The listing builds one solid part. Answer for the finished solid, in the listing's coordinates (mm). Face numbers are marked on the shaded views. A direction names the side the tool comes from. Round coordinates to 2 decimals unless told otherwise and drop trailing zeros. Write each loop counter-clockwise with the first axis right and the second up, starting at its lowest first coordinate (ties: lowest second). Pieces come first, ordered by that corner, then holes. Notation, with made-up numbers: (38.5, 30) - (56.5, 30) arc R15 ccw to (56.5, 58) - close; hole circle Ø4 at (2, 22). An arc over 180 degrees is marked (long way). Return JSON: item names as keys, results as strings. Group by question number.
from build123d import *

# Parameters (mm, degrees)
EXTRUDE_1_DEPTH          = 1
CUT_EXTRUDE_1_DEPTH      = 5
SKETCH_4_R               = 0.4
CUT_EXTRUDE_2_DEPTH      = 5
PATTERN_CIRCULAR_3_COUNT = 3
FILLET_1_R               = 0.4
FILLET_2_R               = 2


with BuildPart() as part:
    # 草图1 → 凸台-拉伸1 (new, symmetric)
    with BuildSketch(Plane(origin=(0, 0, 0), x_dir=(1, 0, 0), z_dir=(0, 1, 0))):
        Polygon((9.041729559, -19.298041681), (-9.041729559, -19.298041681), (-8.175704156, -20.798041681), (8.175704156, -20.798041681), align=None)
        Polygon((2.782050808, -1.818653348), (1.05, -1.818653348), (10.091729559, -17.479388333), (10.957754963, -15.979388333), align=None)
        Polygon((-10.091729559, -17.479388333), (-1.05, -1.818653348), (-2.782050808, -1.818653348), (-10.957754963, -15.979388333), align=None)
        Polygon((-1.05, -6.918653348), (-1.05, -1.818653348), (-10.091729559, -17.479388333), (-5.675, -14.929388333), (-4.625, -16.748041681), (-9.041729559, -19.298041681), (9.041729559, -19.298041681), (4.625, -16.748041681), (5.675, -14.929388333), (10.091729559, -17.479388333), (1.05, -1.818653348), (1.05, -6.918653348), align=None)
    extrude(amount=EXTRUDE_1_DEPTH, both=True)

    # 草图2 → 切除-拉伸1 (cut, symmetric)
    with BuildSketch(Plane(origin=(0, 1, 0), x_dir=(1, 0, 0), z_dir=(0, 1, 0))):
        Polygon((8.591729559, -14.881312122), (2.55, -4.416729559), (2.55, -11.393117934), align=None)
        Polygon((6.041729559, -19.298041681), (0, -15.809847493), (-6.041729559, -19.298041681), align=None)
        Polygon((-2.55, -11.393117934), (-2.55, -4.416729559), (-8.591729559, -14.881312122), align=None)
    extrude(amount=CUT_EXTRUDE_1_DEPTH, both=True, mode=Mode.SUBTRACT)

    # 草图4 → 切除-拉伸2 (cut, symmetric)
    with BuildSketch(Plane(origin=(0, 1, 0), x_dir=(1, 0, 0), z_dir=(0, 1, 0))):
        with Locations((5.475, -15.275798494)):
            Circle(SKETCH_4_R)
        with Locations((4.825, -16.401631519)):
            Circle(SKETCH_4_R)
    cut_extrude_2 = extrude(amount=CUT_EXTRUDE_2_DEPTH, both=True, mode=Mode.SUBTRACT)

    # 阵列(圆周)3: 切除-拉伸2 ×3 about axis
    pattern_circular_3_axis = Axis((-0.013172797, 0, 12.857755803), (0, 1, 0))
    for i in range(1, PATTERN_CIRCULAR_3_COUNT):
        add(cut_extrude_2.rotate(pattern_circular_3_axis, i * 360 / PATTERN_CIRCULAR_3_COUNT), mode=Mode.SUBTRACT)

    # 圆角1
    fillet_1_edges = [part.edges().sort_by_distance(p)[0] for p in [
        (-2.55, 0, 4.416729559),
        (-8.591729559, 0, 14.881312122),
        (-6.041729559, 0, 19.298041681),
        (6.041729559, 0, 19.298041681),
        (8.591729559, 0, 14.881312122),
        (2.55, 0, 4.416729559),
    ]]
    fillet(fillet_1_edges, radius=FILLET_1_R)

    # 圆角2
    fillet_2_edges = [part.edges().sort_by_distance(p)[0] for p in [
        (-2.55, 0, 11.393117934),
        (0, 0, 15.809847493),
        (2.55, 0, 11.393117934),
    ]]
    fillet(fillet_2_edges, radius=FILLET_2_R)


solid = part.part
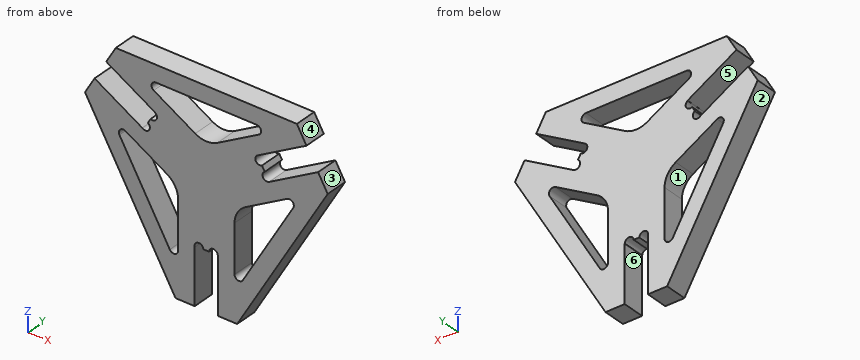
(1) Flat-ended cylindrical pins translate along their axes: pin 1 (1.5 mm diameter, centred on x = -6, z = 5, fed in from -Y); pin 2 (1 mm diameter, centred on y = 0.5, z = 8.5, fed in from +X); pin 3 (1 mm diameter, centred on y = 0, z = 10, fed in from -X); pin 4 (0.6 mm diameter, centred on y = 0, z = 4.5, fed in from +X). Find the tip coordinate at first contact, or state that the pin passes through.
(2) Consider line 1 (Z direction, x = 5.75, y = -0.5); line 2 (X direction, y = -0.6, z = 13.5); line 3 (Z direction, x = 7.5, y = -0.05). Determine where each line is inside the solid, lowest interval first.
(3) For the marked faces 4, 5 and 6, determine the directions among +Z, -Z, +X, -X, +Y, -Y from which every point of the face is accessible in a straight line to the end or side of a thin tool.
(4) Find section A-A (x = 8.75). Write down the section's boundary in (y, z).
(5) Determine the mould class of the marked faces 1, 2 and 3 for opening direction Z: +Z half, -Z half, draft (parallel to the pull), parting line (faces both ways), or undercut.
(6) Find section C-C (z = 9.25). Write down the section's boundary in (x, y).
(7) Find section B-B (x = -4). Write down the section's boundary in (y, z).
(8) Find section D-D (y = -0.7). State how many separate pieces and enclosed holes the cut face has, plus the area to 3 significant figures.
Check sheet entries:
{
 "1": {"pin 1": "passes through", "pin 2": "stops at x = 6.93", "pin 3": "stops at x = -7.79", "pin 4": "stops at x = 4.5"},
 "2": {"line 1": "z = 6.96 to 9.96, 13.24 to 14.97, 17.4 to 20.8", "line 2": "x = -9.53 to -7.79, -6.2 to 6.2, 7.79 to 9.53", "line 3": "z = 9.99 to 12.99, 14.19 to 15.98, 18.41 to 20.8"},
 "3": {"face 4": "+Z, +X, +Y, -Y", "face 5": "+Y, -Y", "face 6": "-Z, +Y, -Y"},
 "4": {"outline": "(-1, 12.16) - (1, 12.16) - (1, 16.7) - (-1, 16.7) - close; (-1, 19.13) - (1, 19.13) - (1, 19.8) - (-1, 19.8) - close"},
 "5": {"face 1": "undercut", "face 2": "-Z half", "face 3": "+Z half"},
 "6": {"outline": "(-7.07, -1) - (-5.34, -1) - (-5.34, 1) - (-7.07, 1) - close; (-2.55, -1) - (2.55, -1) - (2.55, 1) - (-2.55, 1) - close; (5.34, -1) - (7.07, -1) - (7.07, 1) - (5.34, 1) - close"},
 "7": {"outline": "(-1, 3.93) - (1, 3.93) - (1, 6.93) - (-1, 6.93) - close; (-1, 12.23) - (1, 12.23) - (1, 18.12) - (-1, 18.12) - close; (-1, 19.3) - (1, 19.3) - (1, 20.8) - (-1, 20.8) - close"},
 "8": {"separate pieces": "1", "enclosed holes": "3", "area": "193 mm^2"}
}
